from build123d import *

# Parameters (mm, degrees)
SKETCH1_W        = 38.1
SKETCH1_H        = 25.4
EXTRUSION1_DEPTH = 38.1
SHELL1_T         = -3.175
HOLE1_D          = 6.35
SKETCH4_W        = 38.1
SKETCH4_H        = 38.1
SKETCH4_W_2      = 31.75
SKETCH4_H_2      = 31.75
EXTRUSION2_DEPTH = 5.3848
SKETCH5_W        = 38.1
SKETCH5_H        = 5.3848
EXTRUSION3_DEPTH = 38.1


with BuildPart() as part:
    # Sketch1 → Extrusion1 (new body)
    with BuildSketch(Plane(origin=(0, 0, 0), x_dir=(-1, 0, 0), z_dir=(0, 1, 0))):
        Rectangle(SKETCH1_W, SKETCH1_H)
    extrude(amount=EXTRUSION1_DEPTH)

    # Shell1
    shell1_openings = [part.faces().sort_by_distance(p)[0] for p in [
        (0, 19.05, 12.7),
        (0, 19.05, -12.7),
    ]]
    offset(amount=SHELL1_T, openings=shell1_openings, kind=Kind.INTERSECTION)

    # Hole1 (through all)
    with Locations(Plane(origin=(0, 38.1, 0), x_dir=(1, 0, 0), z_dir=(0, 1, 0))):
        with Locations((0, 0)):
            Hole(HOLE1_D / 2)

    # Sketch4 → Extrusion2 (add)
    with BuildSketch(Plane.XY.offset(12.7)):
        with Locations((0, 19.05)):
            Rectangle(SKETCH4_W, SKETCH4_H)
        with Locations((0, 19.05)):
            Rectangle(SKETCH4_W_2, SKETCH4_H_2, mode=Mode.SUBTRACT)
    extrude(amount=EXTRUSION2_DEPTH)

    # Sketch5 → Extrusion3 (cut)
    with BuildSketch(Plane(origin=(0, 38.1, 0), x_dir=(1, 0, 0), z_dir=(0, 1, 0))):
        with Locations((0, -15.3924)):
            Rectangle(SKETCH5_W, SKETCH5_H)
    extrude(amount=-EXTRUSION3_DEPTH, mode=Mode.SUBTRACT)


solid = part.part
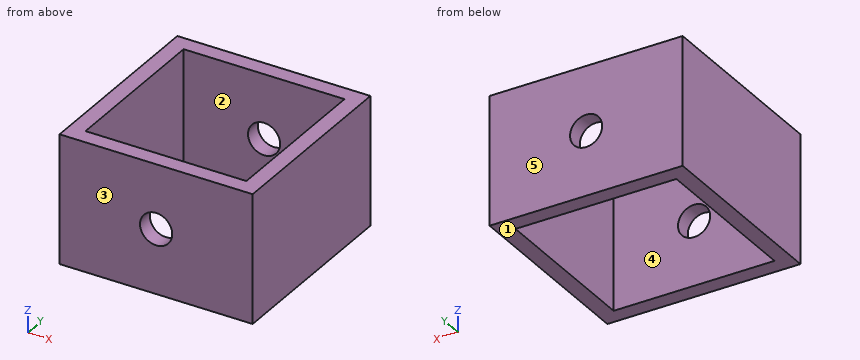
The listing builds one solid part. Answer for the finished solid, in the listing's coordinates (mm). Face numbers are marked on the shaded views. A direction names the side the tool comes from. Coordinates: 2 decimals unless noted, no trailing zeros. Write each loop counter-clockwise with the first axis right and the second up, starting at its lowest first coordinate (ties: lowest second). Pieces come first, ordered by that corner, then holes. Notation, with made-up numbers: (7.25, 31) - (47.25, 31) arc R17 ccw to (47.25, 36) - close; hole circle Ø2 at (87, 74.5). An arc over 180 degrees is marked (long way). Return JSON: item names as keys, results as strings.
1. Consider line 1 along Y through (x, z) = (-15, -6.25) (3 decimals); line 2 along X through (y, z) = (11, -9) (3 decimals); line 3 along Z through (x, y) = (0, 1.15) (3 decimals). Determine where each line is inside the solid, lowest interval first.
Final values:
{"line 1": "0 to 3.175, 34.925 to 38.1", "line 2": "-19.05 to -15.875, 15.875 to 19.05", "line 3": "-12.7 to -3.175, 3.175 to 12.7"}
2. The part is cut by section A-A on y = 9.5. Determine the outline of the cut face in (x, z) (3 decimals).
Final values:
{"outline": "(-19.05, -12.7) - (-15.875, -12.7) - (-15.875, 12.7) - (-19.05, 12.7) - close; (15.875, -12.7) - (19.05, -12.7) - (19.05, 12.7) - (15.875, 12.7) - close"}
3. The part is cut by section D-D on x = 0.5. Determine the outline of the cut face in (y, z) (3 decimals), then the cut area to 3 significant figures.
Final values:
{"outline": "(0, -12.7) - (3.175, -12.7) - (3.175, -3.135) - (0, -3.135) - close; (0, 3.135) - (3.175, 3.135) - (3.175, 12.7) - (0, 12.7) - close; (34.925, -12.7) - (38.1, -12.7) - (38.1, -3.135) - (34.925, -3.135) - close; (34.925, 3.135) - (38.1, 3.135) - (38.1, 12.7) - (34.925, 12.7) - close", "area": "121 mm^2"}
4. Which of the six approach directions +Z, -Z, +X, -X, +Y, -Y give full straight-line access (tool end or side, diameter ignored) to the marked faces 1 and 2?
Final values:
{"face 1": "-Z, +X, -X, +Y, -Y", "face 2": "+Z, -Z"}
5. For a pull along Y with two mould halves and no side action, classify the marked faces 3, 4 and 5 as +Y half, -Y half, draft (parallel to the pull), parting line (faces both ways), or undercut.
Final values:
{"face 3": "-Y half", "face 4": "undercut", "face 5": "+Y half"}
6. The part is cut by section B-B on x = 6.5. Determine the outline of the cut face in (y, z) (3 decimals), then the cut area to 3 significant figures.
Final values:
{"outline": "(0, -12.7) - (3.175, -12.7) - (3.175, 12.7) - (0, 12.7) - close; (34.925, -12.7) - (38.1, -12.7) - (38.1, 12.7) - (34.925, 12.7) - close", "area": "161 mm^2"}
7. The part is cut by section C-C on z = 0. Determine the outline of the cut face in (x, y) (3 decimals).
Final values:
{"outline": "(-19.05, 0) - (-3.175, 0) - (-3.175, 3.175) - (-15.875, 3.175) - (-15.875, 34.925) - (-3.175, 34.925) - (-3.175, 38.1) - (-19.05, 38.1) - close; (3.175, 0) - (19.05, 0) - (19.05, 38.1) - (3.175, 38.1) - (3.175, 34.925) - (15.875, 34.925) - (15.875, 3.175) - (3.175, 3.175) - close"}
